from build123d import *

# Parameters (mm, degrees)
F0_R     = 25
F1_DEPTH = 40
F6_R     = 5


with BuildPart() as f1:
    # F0 (on Top) → F1 (new body)
    with BuildSketch(Plane.XY):
        Circle(F0_R)
    extrude(amount=F1_DEPTH)

    # F4 (on 3pt) → F5 (revolve, cut)
    with BuildSketch(Plane(origin=(0, 0, 0), x_dir=(0.0647328202, 0.9979026315, 0), z_dir=(0.9979026315, -0.0647328202, 0))):
        Polygon((6, 40), (0, 40), (0, 8), align=None)
    revolve(axis=Axis((0, 0, 24), (0, 0, -1)), mode=Mode.SUBTRACT)

    # F6
    f6_edges = [f1.edges().sort_by_distance(p)[0] for p in [
        (-25, 0, 40),
    ]]
    fillet(f6_edges, radius=F6_R)


solid = f1.part
Geometry check sheet. Reference: the model listing, model coordinates, mm. Round coordinates to 2 decimals unless told otherwise and drop trailing zeros. Write each loop counter-clockwise with the first axis right and the second up, starting at its lowest first coordinate (ties: lowest second). Pieces come first, ordered by that corner, then holes. Notation, with made-up numbers: (-27, 61) -> (13, 61) arc R25 cw to (13, 73) -> close; hole circle Ø7 at (53, -30.75). An arc over 180 degrees is marked (long way). One line per item, written item: value. Start each with the question number.
(1) Draft check along Y on faces 1 (the flat face through (4, 5, 40)), 2 (the conical face through (0, -3, 24)), 3 (the cylindrical face through (23.846, 7.509, 17.255)). Enter one of: +Y half, -Y half, draft (parallel to the pull), parting line (faces both ways), or undercut.
(2) Cross-section at A-A, the plane z = 3. Record the cut outline in (x, y), and give its area (3 significant figures).
(3) Go/stop test with flat-tipped pins: pin 1 Ø12 at (x, z) = (17, 7.5) entering from -Y; pin 2 Ø12 at (x, z) = (15.5, 22.5) entering from +Y; pin 3 Ø6 at (y, z) = (-16.5, 19.5) entering from +X. Record where each tip stops, or that it passes through.
(4) Scan lines: line 1 (X direction, y = -6, z = 36); line 2 (Y direction, x = -1, z = 8.5); line 3 (Y direction, x = 2.5, z = 3.5). Record each from-to range of solid material in increasing order. Write a range as [from, to].
Answer:
1. face 1: draft
1. face 2: undercut
1. face 3: parting line
2. outline: circle Ø50 at (0, 0)
2. area: 1,960 mm²
3. pin 1: y = -22.45
3. pin 2: y = 23.12
3. pin 3: x = 21.04
4. line 1: [-24.17, 24.17]
4. line 2: [-24.98, 24.98]
4. line 3: [-24.87, 24.87]
